```python
from build123d import *

# Parameters (mm, degrees)
SKETCH1_W           = 88
SKETCH1_H           = 37
SKETCH1_R           = 1.6
BOSS_EXTRUDE1_DEPTH = 5
FILLET1_R           = 5
CHAMFER2_SIZE       = 1.5
SKETCH2_R           = 1.25
CUT_EXTRUDE1_DEPTH  = 10
SKETCH3_W           = 10
SKETCH3_H           = 10
CUT_EXTRUDE2_DEPTH  = 10
FILLET2_R           = 3


with BuildPart() as part:
    # Sketch1 → Boss-Extrude1 (new body)
    with BuildSketch(Plane.YZ):
        Rectangle(SKETCH1_W, SKETCH1_H)
        with Locations(Location((-41.5, -15.5, 0), (0, 0, 270))):
            Circle(SKETCH1_R, mode=Mode.SUBTRACT)
        with Locations(Location((-41.5, -3, 0), (0, 0, 270))):
            Circle(SKETCH1_R, mode=Mode.SUBTRACT)
        with Locations(Location((41.5, -15.5, 0), (0, 0, 90))):
            Circle(SKETCH1_R, mode=Mode.SUBTRACT)
        with Locations(Location((-26, 14, 0), (0, 0, 270))):
            Circle(SKETCH1_R, mode=Mode.SUBTRACT)
        with Locations(Location((-26, -12, 0), (0, 0, 270))):
            Circle(SKETCH1_R, mode=Mode.SUBTRACT)
        with Locations(Location((41.5, -0.5, 0), (0, 0, 270))):
            Circle(SKETCH1_R, mode=Mode.SUBTRACT)
        with BuildLine():
            Line((-24, -8.2), (-24, 11.8))
            ThreePointArc((-24, 11.8), (-22.86444197, 13.331108636), (-21.069632929, 12.688888889))
            ThreePointArc((-21.069632929, 12.688888889), (-20.349483132, 12.036165793), (-19.406674091, 11.8))
            Line((-19.406674091, 11.8), (26.806674091, 11.8))
            ThreePointArc((26.806674091, 11.8), (27.749483132, 12.036165793), (28.469632929, 12.688888889))
            ThreePointArc((28.469632929, 12.688888889), (30.26444197, 13.331108636), (31.4, 11.8))
            Line((31.4, 11.8), (31.4, -8.2))
            ThreePointArc((31.4, -8.2), (30.26444197, -9.731108636), (28.469632929, -9.088888889))
            ThreePointArc((28.469632929, -9.088888889), (27.749483132, -8.436165793), (26.806674091, -8.2))
            Line((26.806674091, -8.2), (-19.406674091, -8.2))
            ThreePointArc((-19.406674091, -8.2), (-20.349483132, -8.436165793), (-21.069632929, -9.088888889))
            ThreePointArc((-21.069632929, -9.088888889), (-22.86444197, -9.731108636), (-24, -8.2))
        make_face(mode=Mode.SUBTRACT)
    extrude(amount=BOSS_EXTRUDE1_DEPTH)

    # Fillet1
    fillet1_edges = [part.edges().sort_by_distance(p)[0] for p in [
        (2.5, -44, 18.5),
        (2.5, 44, 18.5),
    ]]
    fillet(fillet1_edges, radius=FILLET1_R)

    # Chamfer2
    # the kernel refuses this chamfer: 1.5 mm, written as the material it takes off along each edge
    with BuildSketch(Plane(origin=(5, -41.5, -15.5), x_dir=(0, 0, -1), z_dir=(0, -1, 0))) as chamfer2_piece_1:
        Polygon((1.6 + CHAMFER2_SIZE, 0), (1.6, -CHAMFER2_SIZE), (1.6, 0), align=None)
    revolve(axis=Axis((5, -41.5, -15.5), (1, 0, 0)), mode=Mode.SUBTRACT)
    with BuildSketch(Plane(origin=(5, -41.5, -3), x_dir=(0, 0, -1), z_dir=(0, -1, 0))) as chamfer2_piece_2:
        Polygon((1.6 + CHAMFER2_SIZE, 0), (1.6, -CHAMFER2_SIZE), (1.6, 0), align=None)
    revolve(axis=Axis((5, -41.5, -3), (1, 0, 0)), mode=Mode.SUBTRACT)
    with BuildSketch(Plane(origin=(5, 41.5, -0.5), x_dir=(0, 0, -1), z_dir=(0, -1, 0))) as chamfer2_piece_3:
        Polygon((1.6 + CHAMFER2_SIZE, 0), (1.6, -CHAMFER2_SIZE), (1.6, 0), align=None)
    revolve(axis=Axis((5, 41.5, -0.5), (1, 0, 0)), mode=Mode.SUBTRACT)
    with BuildSketch(Plane(origin=(5, 41.5, -15.5), x_dir=(0, 0, 1), z_dir=(0, 1, 0))) as chamfer2_piece_4:
        Polygon((1.6 + CHAMFER2_SIZE, 0), (1.6, -CHAMFER2_SIZE), (1.6, 0), align=None)
    revolve(axis=Axis((5, 41.5, -15.5), (1, 0, 0)), mode=Mode.SUBTRACT)
    with BuildSketch(Plane(origin=(5, -26, 14), x_dir=(0, 0, -1), z_dir=(0, -1, 0))) as chamfer2_piece_5:
        Polygon((1.6 + CHAMFER2_SIZE, 0), (1.6, -CHAMFER2_SIZE), (1.6, 0), align=None)
    revolve(axis=Axis((5, -26, 14), (1, 0, 0)), mode=Mode.SUBTRACT)
    with BuildSketch(Plane(origin=(5, -26, -12), x_dir=(0, 0, -1), z_dir=(0, -1, 0))) as chamfer2_piece_6:
        Polygon((1.6 + CHAMFER2_SIZE, 0), (1.6, -CHAMFER2_SIZE), (1.6, 0), align=None)
    revolve(axis=Axis((5, -26, -12), (1, 0, 0)), mode=Mode.SUBTRACT)

    # Sketch2 → Cut-Extrude1 (cut)
    with BuildSketch(Plane.YZ.offset(5)):
        with Locations(Location((-36.826603685, -0.023130638, 0), (0, 0, 270))):
            Circle(SKETCH2_R)
        with Locations(Location((-33.167413509, -14.120748425, 0), (0, 0, 270))):
            Circle(SKETCH2_R)
        with Locations(Location((33.182572395, -14.077498807, 0), (0, 0, 270))):
            Circle(SKETCH2_R)
    extrude(amount=-CUT_EXTRUDE1_DEPTH, mode=Mode.SUBTRACT)

    # Sketch3 → Cut-Extrude2 (cut)
    with BuildSketch(Plane.YZ.offset(5)):
        with Locations((-39, 13.5)):
            Rectangle(SKETCH3_W, SKETCH3_H)
        with Locations((39, 13.5)):
            Rectangle(SKETCH3_W, SKETCH3_H)
    extrude(amount=-CUT_EXTRUDE2_DEPTH, mode=Mode.SUBTRACT)

    # Fillet2
    fillet2_edges = [part.edges().sort_by_distance(p)[0] for p in [
        (2.5, -34, 18.5),
        (2.5, -34, 8.5),
        (2.5, -44, 8.5),
        (2.5, 44, 8.5),
        (2.5, 34, 8.5),
        (2.5, 34, 18.5),
    ]]
    fillet(fillet2_edges, radius=FILLET2_R)


solid = part.part
```
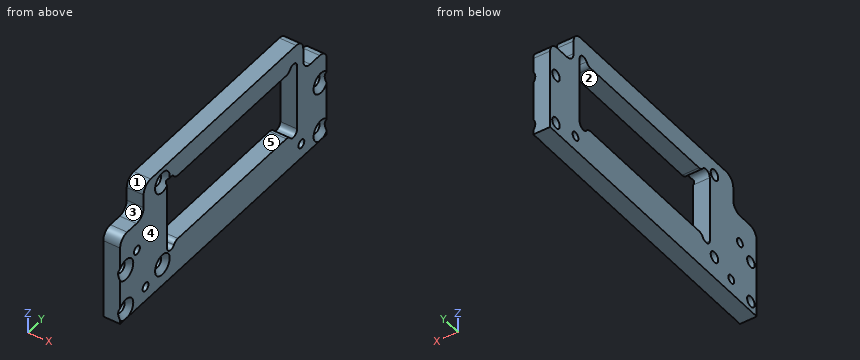
Source: CAD feature listing. Evaluate the final solid. Frame: model axes, mm. Face numbers are marked on the shaded views. A direction names the side the tool comes from. Give positions to 0.01 mm unless a question says otherwise; leave off trailing zeros. Loops run counter-clockwise (first coordinate to the right, second up) from the corner with the lowest first, then second, coordinate; pieces in that order, holes last. Notation, with made-up numbers: (-35.75, 60.25) - (15.25, 60.25) arc R23 ccw to (15.25, 75.25) - close; hole circle Ø2 at (-30, -20). An arc over 180 degrees is marked (long way). Use CSV: the item, a comma, the result in double quotes.
1) Line query: line 1 (Y direction, x = 0.8, z = 14); line 2 (Z direction, x = 4.45, y = 22.5); line 3 (Y direction, x = 4.7, z = 3). Output: solid intervals per line, ascending.
Worked out:
line 1,"y = -34 to -27.6, -24.4 to 34"
line 2,"z = -18.5 to -8.2, 11.8 to 18.5"
line 3,"y = -44 to -24, 31.4 to 44"
2) Cut plane B-B (z = 9.5). Output: boundary loops of the cut face in (x, y).
Worked out:
outline,"(0, -34.76) - (5, -34.76) - (5, -24) - (0, -24) - close; (0, 31.4) - (5, 31.4) - (5, 34.76) - (0, 34.76) - close"
3) Mould query, pull axis Y, two halves, no side actions, for the marked faces 3, 4 and 5. Classes: +Y half, -Y half, draft (parallel to the pull), parting line (faces both ways), or undercut.
Worked out:
face 3,"-Y half"
face 4,"draft"
face 5,"undercut"
4) Pin query (flat end, axial travel): P1, Ø3.5, axis at y = -41.5, z = -3, coming from the +X side; P2, Ø2, axis at y = -33.17, z = -14.12, coming from the +X side; P3, Ø1.2, axis at x = 2, y = -39, coming from the +Z side; P4, Ø5, axis at y = -22.5, z = 9.5, coming from the +X side. Return the tip coordinate at first contact, or that it passes through.
Worked out:
P1,"stops at x = 3.65"
P2,"passes through"
P3,"stops at z = 8.5"
P4,"stops at x = 5"
5) Set-up query: the marked faces 1 and 2. Return all of +Z, -Z, +X, -X, +Y, -Y with unobstructed straight access to the full face (end or side cutting, diameter ignored); none if empty.
Worked out:
face 1,"+Z, +X, -X, -Y"
face 2,"+X, -X"
6) Cut plane A-A (y = 16). Output: boundary loops of the cut face in (x, z), and give its area (3 significant figures).
Worked out:
outline,"(0, -18.5) - (5, -18.5) - (5, -8.2) - (0, -8.2) - close; (0, 11.8) - (5, 11.8) - (5, 18.5) - (0, 18.5) - close"
area,"85.0 mm^2"
